Check sheet for the modelled part. Datum: model origin and axes. Units: mm. A direction names the side the tool comes from. Coordinates: 2 decimals unless noted, no trailing zeros. Order: outer loops, then holes, each group sorted by start corner. A loop starts at its lowest first (then second) coordinate and runs counter-clockwise, first axis right, second up. Notation, with made-up numbers: (55, -11) -> (81, -11) arc R28 cw to (81, 20) -> close; hole circle Ø7 at (11.5, 15.25). An arc over 180 degrees is marked (long way). Put each result on its own line as item: value. Start each with the question number.
```python
from build123d import *

# Parameters (mm, degrees)
F0_W      = 101.6
F0_H      = 12.7
F1_DEPTH  = 25.4
F2_R      = 6.35
F3_DEPTH  = 25.4
F4_R      = 9.525
F5_DEPTH  = 38.1
F6_R      = 6.35
F7_DEPTH  = 50.8
F9_DEPTH  = 25.4
F11_DEPTH = 25.4
F13_DEPTH = 25.4


with BuildPart() as f1:
    # F0 (on Front) → F1 (new body)
    with BuildSketch(Plane.XZ):
        with Locations((50.8, 6.35)):
            Rectangle(F0_W, F0_H)
    extrude(amount=F1_DEPTH)

    # F2 (on face) → F3 (cut)
    with BuildSketch(Plane.XY.offset(12.7)):
        with Locations((12.7, -12.7)):
            Circle(F2_R)
    extrude(amount=-F3_DEPTH, mode=Mode.SUBTRACT)

    # F4 (on face) → F5 (join)
    with BuildSketch(Plane.XY.offset(12.7)):
        with Locations((30.8962874115, -12.7)):
            Circle(F4_R)
    extrude(amount=F5_DEPTH)

    # F6 (on face) → F7 (cut)
    with BuildSketch(Plane.XY.offset(50.8)):
        with Locations((30.8962874115, -12.7)):
            Circle(F6_R)
    extrude(amount=-F7_DEPTH, mode=Mode.SUBTRACT)

    # F8 (on face) → F9 (cut)
    with BuildSketch(Plane.XY.offset(12.7)):
        with BuildLine():
            ThreePointArc((61.5597656887, -12.7), (59.6998937492, -17.1901280605), (55.2097656887, -19.05))
            Line((55.2097656887, -19.05), (77.399272464, -18.8575478586))
            ThreePointArc((77.399272464, -18.8575478586), (72.6114019876, -12.3324709451), (78.1212527055, -6.4044124523))
            Line((78.1212527055, -6.4044124523), (56.0392700164, -6.4044124523))
            ThreePointArc((56.0392700164, -6.4044124523), (59.9841689227, -8.5134054699), (61.5597656887, -12.7))
        make_face()
        with BuildLine():
            Line((56.0392700164, -6.4044124523), (54.3802613609, -6.4044124523))
            ThreePointArc((54.3802613609, -6.4044124523), (48.8733834035, -13.1156435206), (55.2097656887, -19.05))
            ThreePointArc((55.2097656887, -19.05), (59.6998937492, -17.1901280605), (61.5597656887, -12.7))
            ThreePointArc((61.5597656887, -12.7), (59.9841689227, -8.5134054699), (56.0392700164, -6.4044124523))
        make_face()
        with BuildLine():
            ThreePointArc((78.1212527055, -6.4044124523), (72.6114019876, -12.3324709451), (77.399272464, -18.8575478586))
            Line((77.399272464, -18.8575478586), (80.6088104115, -18.8297111673))
            ThreePointArc((80.6088104115, -18.8297111673), (83.9931343967, -16.5596541975), (85.3007570332, -12.7))
            ThreePointArc((85.3007570332, -12.7), (83.7251602672, -8.5134054699), (79.7802613609, -6.4044124523))
            Line((79.7802613609, -6.4044124523), (78.1212527055, -6.4044124523))
        make_face()
    extrude(amount=-F9_DEPTH, mode=Mode.SUBTRACT)

    # F10 (on face) → F11 (cut)
    with BuildSketch(Plane.XY.offset(12.7)):
        with BuildLine():
            ThreePointArc((76.106920933, 0), (88.806920933, -12.7), (76.106920933, -25.4))
            Line((76.106920933, -25.4), (101.6, -25.4))
            Line((101.6, -25.4), (101.6, 0))
            Line((101.6, 0), (76.106920933, 0))
        make_face()
    extrude(amount=-F11_DEPTH, mode=Mode.SUBTRACT)

    # F12 (on face) → F13 (cut)
    with BuildSketch(Plane.XY.offset(12.7)):
        with BuildLine():
            ThreePointArc((14.8660039439, -25.4), (2.1660039439, -12.7), (14.8660039439, 0))
            Line((14.8660039439, 0), (0, 0))
            Line((0, 0), (0, -25.4))
            Line((0, -25.4), (14.8660039439, -25.4))
        make_face()
    extrude(amount=-F13_DEPTH, mode=Mode.SUBTRACT)


solid = f1.part
```
1) Sectioned sample at A-A (z = 47). Record the boundary of the cut face in (x, y) (3 decimals), plus the area to 3 significant figures.
2) Scan lines: line 1 along X through (y, z) = (-7.5, 36); line 2 along X through (y, z) = (-17, 23.5); line 3 along Y through (x, z) = (31.5, 7.5). Record each from-to range of solid material in increasing order. Write a range as [from, to].
3) Access from +Z, -Z, +X, -X, +Y, -Y to the whole of each face (thin tool, end or side, straight path). Record for faces 5 (the cylindrical face through (39.98, -9.84, 31.48)), 6 (the cylindrical face through (88.804, -12.421, 6.439)).
4) Mould release check, pull along Y, two halves, no side actions. Record for faces 1 (the flat face through (33, -19, 50.8)), 2 (the flat face through (45, 0, 6)), 3 (the flat face through (67, -6.404, 6)), 4 (the cylindrical face through (33.83, -18.33, 25.76)): +Y half, -Y half, draft (parallel to the pull), parting line (faces both ways), or undercut.
5) Sectioned sample at B-B (x = 12.7). Record the boundary of the cut face in (y, z).
6) Gauge pin test, flat ends, axial feed: pin 1 (10 mm diameter, centred on x = 64.5, y = -6.5, fed in from +Z); pin 2 (6 mm diameter, centred on y = -21.5, z = 31, fed in from -X); pin 3 (2 mm diameter, centred on x = 26, z = 35, fed in from -Y). Record the tip position at first contact, or that the pin passes through.
7) Sectioned sample at C-C (y = -1.5). Record the boundary of the cut face in (x, z), plus the area to 3 significant figures.
Entries:
1. outline: circle Ø19.05 at (30.896, -12.7); hole circle Ø12.7 at (30.896, -12.7)
1. area: 158 mm2
2. line 1: x = [22.92, 27.25], [34.54, 38.88]
2. line 2: x = [22.4, 26.22], [35.57, 39.4]
2. line 3: y = [-25.4, -19.02], [-6.38, 0]
3. face 5: +Z
3. face 6: +Z, -Z, +X
4. face 1: draft
4. face 2: +Y half
4. face 3: undercut
4. face 4: undercut
5. outline: (-25.21, 0) -> (-19.05, 0) -> (-19.05, 12.7) -> (-25.21, 12.7) -> close; (-6.35, 0) -> (-0.19, 0) -> (-0.19, 12.7) -> (-6.35, 12.7) -> close
6. pin 1: stops at z = 12.7
6. pin 2: stops at x = 23.34
6. pin 3: stops at y = -21.39
7. outline: (8.88, 0) -> (82.09, 0) -> (82.09, 12.7) -> (8.88, 12.7) -> close
7. area: 930 mm2
